Geometry: see drawing. Coordinates: mm, zero at the bounding-box minimum. A direction names the side the tool comes from. Give positions to 0.01 mm unless a question says otherwise; leave off trailing zeros. Write each loop counter-clockwise with the first axis right and the second up, starting at its lowest first coordinate (ties: lowest second). Pieces come first, ordered by that corner, then holes. Notation, with made-up numbers: (48.5, 45) - (93.5, 45) arc R24 ccw to (93.5, 66) - close; hole circle Ø7 at (-25, -37). An arc over 180 degrees is marked (long way). Use a Markdown table: item, result. Add a question column.
1. Section query D-D, the plane z = 22.5. Return loops of the section in (x, y).
2. Material intervals for probe 1 along X at (y, z) = (1, 27); probe 2 along Z at (x, y) = (19, 4); probe 3 along Z at (x, y) = (66, 10.25), sorted ascending.
3. Section query C-C, the plane x = 69.5. Return loops of the section in (y, z), plus the area to 3 significant figures.
4. Pin query (flat end, axial travel): pin 1 (1 mm diameter, centred on y = 18, z = 33, fed in from +X); pin 2 (11 mm diameter, centred on x = 33, y = 9.5, fed in from +Z). Return the tip coordinate at first contact, or that it passes through.
5. Mould query, pull axis Y, two halves, no side actions, for the marked faces 3, 4 and 5. Classes: released by +Y, released by -Y, zero draft, split by the parting line, or undercut.
6. Section query A-A, the plane z = 8. Return loops of the section in (x, y), plus the area to 3 significant figures.
7. Section query B-B, the plane y = 10. Return loops of the section in (x, z), plus the area to 3 significant figures.
8. Set-up query: the marked faces 1 and 2. Return all of +Z, -Z, +X, -X, +Y, -Y with unobstructed straight access to the full face (end or side cutting, diameter ignored); none if empty.
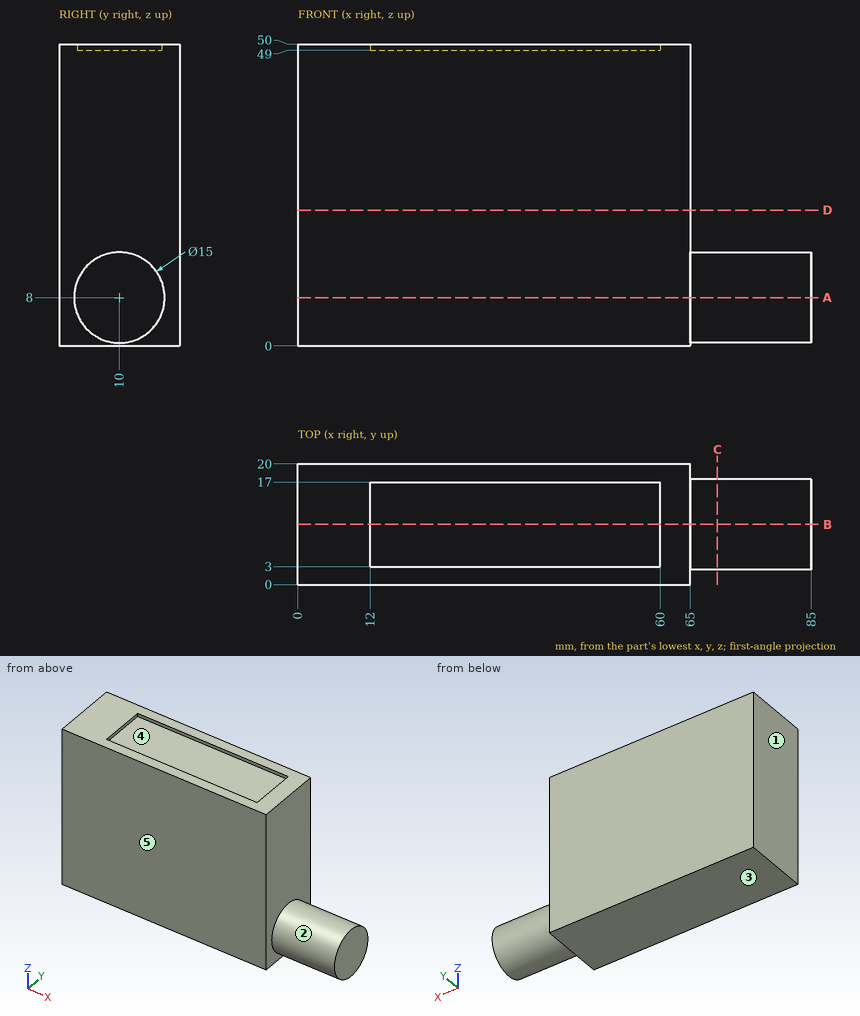
Result sheet:
| question | item | result |
|---|---|---|
| 1 | outline | (0, 0) - (65, 0) - (65, 20) - (0, 20) - close |
| 2 | probe 1 | x = 0 to 65 |
| 2 | probe 2 | z = 0 to 49 |
| 2 | probe 3 | z = 0.5 to 15.5 |
| 3 | outline | circle Ø15 at (10, 8) |
| 3 | area | 177 mm² |
| 4 | pin 1 | stops at x = 65 |
| 4 | pin 2 | stops at z = 49 |
| 5 | face 3 | zero draft |
| 5 | face 4 | undercut |
| 5 | face 5 | released by -Y |
| 6 | outline | (0, 0) - (65, 0) - (65, 2.5) - (85, 2.5) - (85, 17.5) - (65, 17.5) - (65, 20) - (0, 20) - close |
| 6 | area | 1,600 mm² |
| 7 | outline | (0, 0) - (65, 0) - (65, 0.5) - (85, 0.5) - (85, 15.5) - (65, 15.5) - (65, 50) - (60, 50) - (60, 49) - (12, 49) - (12, 50) - (0, 50) - close |
| 7 | area | 3,500 mm² |
| 8 | face 1 | +Z, -Z, -X, +Y, -Y |
| 8 | face 2 | +X |
